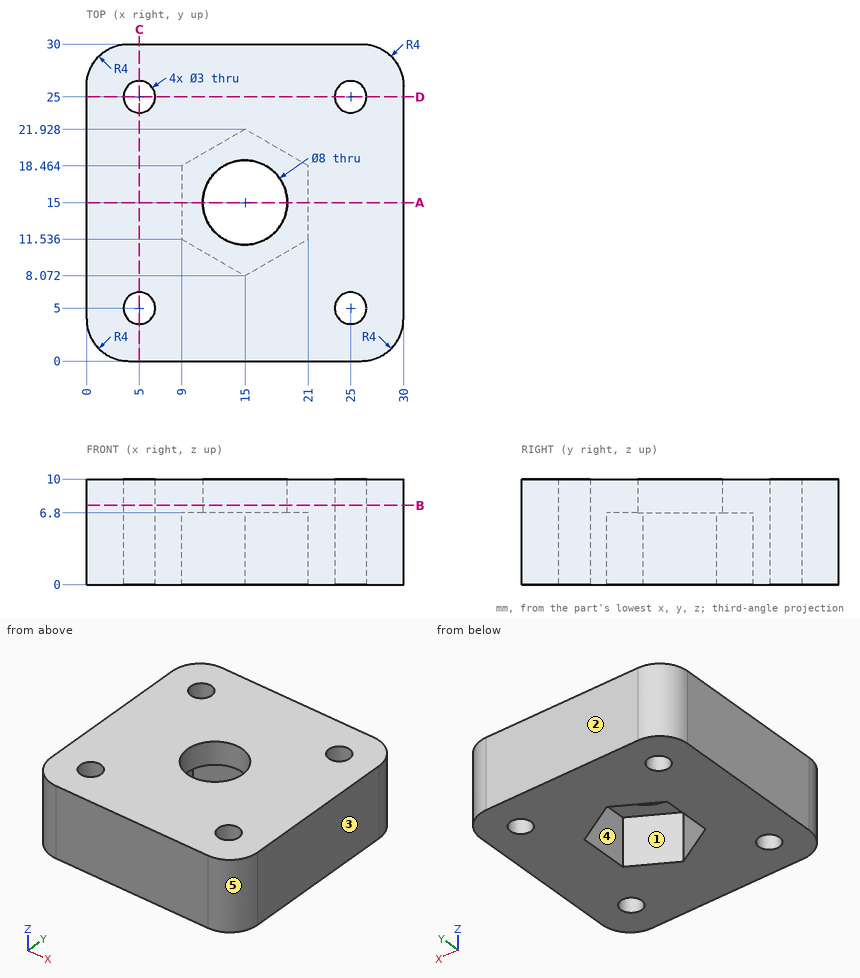
The figure shows three views and two pictorial views of one solid part (mm, origin at its lowest corner). Answer the questions. A direction names the side the tool comes from. Coordinates: 2 decimals unless noted, no trailing zeros. Loops run counter-clockwise (first coordinate to the right, second up) from the corner with the lowest first, then second, coordinate; pieces in that order, holes last. Notation, with made-up numbers: (-20.5, 67) - (24.5, 67) arc R25 cw to (24.5, 87) - close; hole circle Ø11 at (-37.75, 41). An arc over 180 degrees is marked (long way). Use a Markdown table: item, result. Add a question column.
1) The mould has two halves that part along Y. Classify the marked faces 1, 2 and 3: released by +Y, released by -Y, zero draft, split by the parting line, or undercut.
2) The part is cut by section A-A, the plane y = 15. Give the vertices of the cut face in (x, z), and give its area (3 significant figures).
3) Find the intervals of material crossed by line 1 (Y direction, x = 5, z = 3.25); line 2 (Y direction, x = 15, z = 9.15); line 3 (Y direction, x = 4.25, z = 2.25), in increasing order.
4) For the marked faces 4 and 5, determine the directions among +Z, -Z, +X, -X, +Y, -Y from which every point of the face is accessible in a straight line to the end or side of a thin tool.
5) The part is cut by section B-B, the plane z = 7.5. Give the vertices of the cut face in (x, y).
6) Given pin 1 (6 mm diameter, centred on x = 11, y = 9.5, fed in from -Z); pin 2 (6 mm diameter, centred on x = 16, y = 12.5, fed in from -Z), each flat-ended and moving along its own axis, determine where each tip first touches the part or whether it passes through.
7) The part is cut by section C-C, the plane x = 5. Give the vertices of the cut face in (y, z), and give its area (3 significant figures).
Here are the results:
| question | item | result |
|---|---|---|
| 1 | face 1 | undercut |
| 1 | face 2 | released by +Y |
| 1 | face 3 | zero draft |
| 2 | outline | (0, 0) - (9, 0) - (9, 6.8) - (11, 6.8) - (11, 10) - (0, 10) - close; (19, 6.8) - (21, 6.8) - (21, 0) - (30, 0) - (30, 10) - (19, 10) - close |
| 2 | area | 193 mm^2 |
| 3 | line 1 | y = 0 to 3.5, 6.5 to 23.5, 26.5 to 30 |
| 3 | line 2 | y = 0 to 11, 19 to 30 |
| 3 | line 3 | y = 0 to 3.7, 6.3 to 23.7, 26.3 to 30 |
| 4 | face 4 | -Z |
| 4 | face 5 | +Z, -Z, +X, -Y |
| 5 | outline | (0, 4) arc R4 ccw to (4, 0) - (26, 0) arc R4 ccw to (30, 4) - (30, 26) arc R4 ccw to (26, 30) - (4, 30) arc R4 ccw to (0, 26) - close; hole circle Ø3 at (5, 5); hole circle Ø3 at (5, 25); hole circle Ø8 at (15, 15); hole circle Ø3 at (25, 5); hole circle Ø3 at (25, 25) |
| 6 | pin 1 | stops at z = 0 |
| 6 | pin 2 | stops at z = 6.8 |
| 7 | outline | (0, 0) - (3.5, 0) - (3.5, 10) - (0, 10) - close; (6.5, 0) - (23.5, 0) - (23.5, 10) - (6.5, 10) - close; (26.5, 0) - (30, 0) - (30, 10) - (26.5, 10) - close |
| 7 | area | 240 mm^2 |
